from build123d import *

# Parameters (mm, degrees)
SKETCH2_W           = 40
SKETCH2_H           = 20
SKETCH2_R           = 2.665211454
BOSS_EXTRUDE1_DEPTH = 40.5
BOSS_EXTRUDE3_START = 27.8
SKETCH2_5_W         = 7.25
SKETCH2_5_H         = 20
SKETCH2_5_R         = 2.5
BOSS_EXTRUDE3_DEPTH = 6
SKETCH2_6_R         = 2.665211454
BOSS_EXTRUDE4_DEPTH = 45.5


with BuildPart() as part:
    # Sketch2 → Boss-Extrude1 (new body)
    # profile 1 of 2: a face of its own
    with BuildSketch(Plane(origin=(0, 0, 0), x_dir=(1, 0, 0), z_dir=(0, 1, 0))):
        Rectangle(SKETCH2_W, SKETCH2_H)
        with Locations((10, 0)):
            Circle(SKETCH2_R, mode=Mode.SUBTRACT)
    # profile 2 of 2: a face of its own
    with BuildSketch(Plane(origin=(0, 0, 0), x_dir=(1, 0, 0), z_dir=(0, 1, 0))):
        with Locations((10, 0)):
            Circle(SKETCH2_R)
    extrude(amount=BOSS_EXTRUDE1_DEPTH)

    # Sketch2_5 → Boss-Extrude3 (add)
    # profile 1 of 2: a face of its own
    with BuildSketch(Plane(origin=(0, 0, 0), x_dir=(1, 0, 0), z_dir=(0, 1, 0)).offset(BOSS_EXTRUDE3_START)):
        with Locations((-23.625, 0)):
            Rectangle(SKETCH2_5_W, SKETCH2_5_H)
        with Locations(Location((-24.74, -5, 0), (0, 0, 270))):
            Circle(SKETCH2_5_R, mode=Mode.SUBTRACT)
        with Locations(Location((-24.74, 5, 0), (0, 0, 270))):
            Circle(SKETCH2_5_R, mode=Mode.SUBTRACT)
    # profile 2 of 2: a face of its own
    with BuildSketch(Plane(origin=(0, 0, 0), x_dir=(1, 0, 0), z_dir=(0, 1, 0)).offset(BOSS_EXTRUDE3_START)):
        with Locations((23.625, 0)):
            Rectangle(SKETCH2_5_W, SKETCH2_5_H)
        with Locations(Location((24.74, -5, 0), (0, 0, 270))):
            Circle(SKETCH2_5_R, mode=Mode.SUBTRACT)
        with Locations(Location((24.74, 5, 0), (0, 0, 270))):
            Circle(SKETCH2_5_R, mode=Mode.SUBTRACT)
    extrude(amount=BOSS_EXTRUDE3_DEPTH)

    # Sketch2_6 → Boss-Extrude4 (add)
    with BuildSketch(Plane(origin=(0, 0, 0), x_dir=(1, 0, 0), z_dir=(0, 1, 0))):
        with Locations(Location((10, 0, 0), (0, 0, 270))):
            Circle(SKETCH2_6_R)
    extrude(amount=BOSS_EXTRUDE4_DEPTH)


solid = part.part
Geometry: final body of the model. Coordinates: model frame, mm. A direction names the side the tool comes from. Give positions to 0.01 mm unless a question says otherwise; leave off trailing zeros. Write each loop counter-clockwise with the first axis right and the second up, starting at its lowest first coordinate (ties: lowest second). Pieces come first, ordered by that corner, then holes.
(1) Cut plane B-B, the plane z = -8.5. Return loops of the section in (x, y), then the cut area to 3 significant figures.
(2) Cut plane A-A, the plane y = 31.5. Return loops of the section in (x, z).
(3) First-contact query: P1, Ø3, axis at x = -24.74, z = 5, coming from the +Y side; P2, Ø2, axis at x = 22.5, z = -3.5, coming from the -Y side; P3, Ø5, axis at x = -21.5, z = -7, coming from the -Y side; P4, Ø4, axis at x = 19, z = -6, coming from the +Y side. Flat tips, straight axial feed; report the tip coordinate or a pass-through.
(4) Cut plane C-C, the plane z = -5. Give the number of separate pieces and of enclosed holes in the cut face, then the cut area to 3 significant figures.
(5) Access query for faces 5 (the flat face through (24, 33.8, 0)), 6 (the flat face through (-20, 37, 0)), 7 (the cylindrical face through (12.643, 42.965, -0.347)), 8 (the flat face through (-24, 27.8, 0)), 9 (the flat face through (24, 27.8, 0)). Directions: +Z, -Z, +X, -X, +Y, -Y. A direction counts if a zero-diameter tool reaches every point of the face in a straight line with its end or side. Return the directions, or none.
(6) Cut plane D-D, the plane x = 10. Return loops of the section in (y, z).
(7) Mould query, pull axis X, two halves, no side actions, for faces 1 (the cylindrical face through (-22.63, 30.76, -3.66)), 2 (the flat face through (27.25, 31, 0)), 3 (the flat face through (0, 20, 10)), 4 (the cylindrical face through (26.85, 30.76, -3.66)). Classes: released by +X, released by -X, zero draft, split by the parting line, or undercut.
(8) Ray query, line 1 (Y direction, x = -16, z = -1); line 2 (X direction, y = 36.5, z = 0.5). Return the intervals inside material, ascending.
Values follow:
1. outline: (-27.25, 27.8) - (-20, 27.8) - (-20, 0) - (20, 0) - (20, 27.8) - (27.25, 27.8) - (27.25, 33.8) - (20, 33.8) - (20, 40.5) - (-20, 40.5) - (-20, 33.8) - (-27.25, 33.8) - close
1. area: 1,710 mm2
2. outline: (-27.25, -10) - (27.25, -10) - (27.25, 10) - (-27.25, 10) - close; hole circle Ø5 at (-24.74, -5); hole circle Ø5 at (-24.74, 5); hole circle Ø5 at (24.74, -5); hole circle Ø5 at (24.74, 5)
3. P1: passes through
3. P2: stops at y = 27.8
3. P3: stops at y = 0
3. P4: stops at y = 40.5
4. separate pieces: 3
4. enclosed holes: 0
4. area: 1,650 mm2
5. face 5: +Z, -Z, +X, +Y
5. face 6: +Z, -Z, -X, +Y
5. face 7: +Y
5. face 8: +Z, -Z, -X, -Y
5. face 9: +Z, -Z, +X, -Y
6. outline: (0, -10) - (40.5, -10) - (40.5, -2.67) - (45.5, -2.67) - (45.5, 2.67) - (40.5, 2.67) - (40.5, 10) - (0, 10) - close
7. face 1: undercut
7. face 2: released by +X
7. face 3: zero draft
7. face 4: undercut
8. line 1: y = 0 to 40.5
8. line 2: x = -20 to 20
